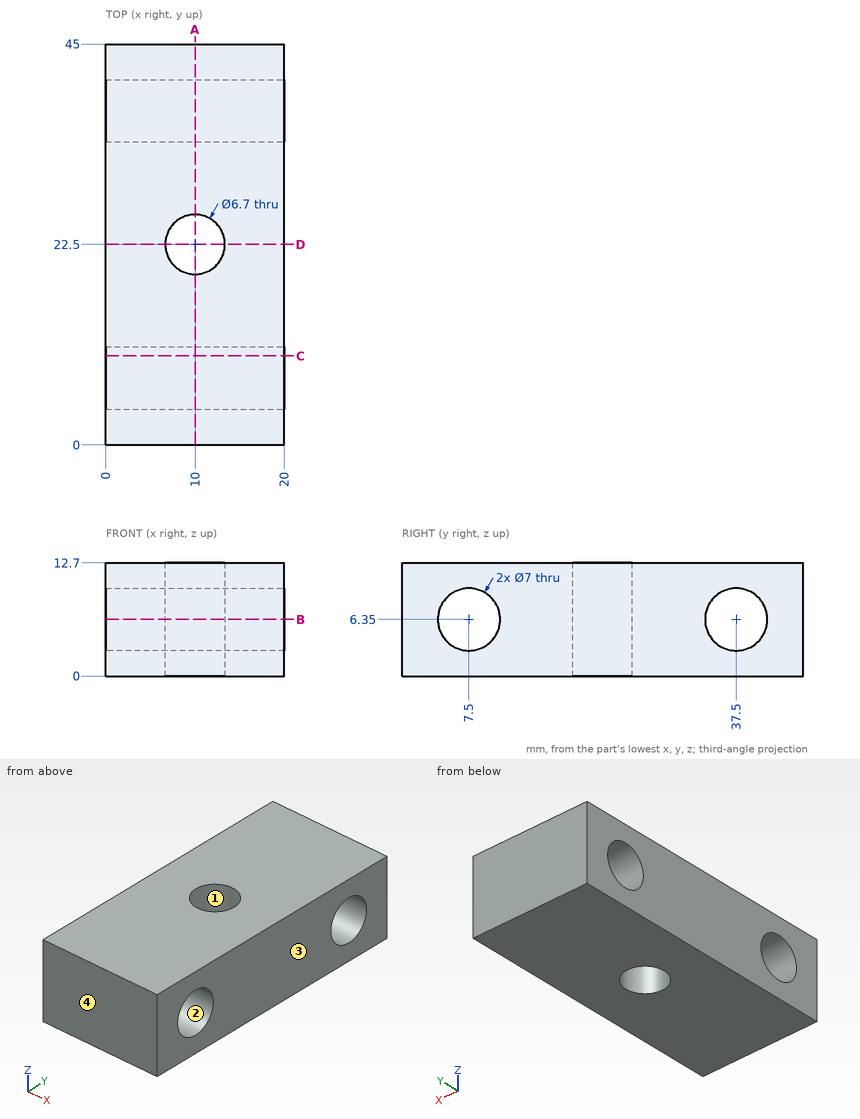
Drawing for the job (mm, zero at the part's lowest x, y, z). Give positions to 0.01 mm unless a question says otherwise; leave off trailing zeros. Loops run counter-clockwise (first coordinate to the right, second up) from the corner with the lowest first, then second, coordinate; pieces in that order, holes last.
1) Band-saw the part on C-C on y = 10. List the corners of the cut face in (x, z).
Values follow:
outline: (0, 0) - (20, 0) - (20, 3.9) - (0, 3.9) - close; (0, 8.8) - (20, 8.8) - (20, 12.7) - (0, 12.7) - close
2) Band-saw the part on B-B on z = 6.35. List the corners of the cut face in (x, y).
Values follow:
outline: (0, 0) - (20, 0) - (20, 4) - (0, 4) - close; (0, 11) - (20, 11) - (20, 34) - (0, 34) - close; (0, 41) - (20, 41) - (20, 45) - (0, 45) - close; hole circle Ø6.7 at (10, 22.5)
3) Band-saw the part on A-A on x = 10. List the corners of the cut face in (y, z), then the cut area to 3 significant figures.
Values follow:
outline: (0, 0) - (19.15, 0) - (19.15, 12.7) - (0, 12.7) - close; (25.85, 0) - (45, 0) - (45, 12.7) - (25.85, 12.7) - close; hole circle Ø7 at (7.5, 6.35); hole circle Ø7 at (37.5, 6.35)
area: 409 mm2
4) Probe line 1 along Y through (x, z) = (6.5, 6.35); line 2 along Y through (x, z) = (10, 6.35); line 3 along Y through (x, z) = (10.75, 4.75). List the from-to ranges inside material, lowest first.
Values follow:
line 1: y = 0 to 4, 11 to 34, 41 to 45
line 2: y = 0 to 4, 11 to 19.15, 25.85 to 34, 41 to 45
line 3: y = 0 to 4.39, 10.61 to 19.24, 25.76 to 34.39, 40.61 to 45
5) Band-saw the part on D-D on y = 22.5. List the corners of the cut face in (x, z), then the cut area to 3 significant figures.
Values follow:
outline: (0, 0) - (6.65, 0) - (6.65, 12.7) - (0, 12.7) - close; (13.35, 0) - (20, 0) - (20, 12.7) - (13.35, 12.7) - close
area: 169 mm2
6) Two-plate mould, pull along Y, no slides. Class the marked faces 1, 2, 3 and 4: released by +Y, released by -Y, zero draft, split by the parting line, or undercut.
Values follow:
face 1: undercut
face 2: undercut
face 3: zero draft
face 4: released by -Y
